Geometry: final body of the model. Coordinates: model frame, mm. A direction names the side the tool comes from. Give positions to 0.01 mm unless a question says otherwise; leave off trailing zeros. Loops run counter-clockwise (first coordinate to the right, second up) from the corner with the lowest first, then second, coordinate; pieces in that order, holes last.
```python
from build123d import *

# Parameters (mm, degrees)
CROQUIS2_R              = 6.5
SALIENTE_EXTRUIR1_DEPTH = 3
CROQUIS3_R              = 3
SALIENTE_EXTRUIR2_DEPTH = 70
CROQUIS4_OUTSIDE_W      = 32.968
CROQUIS4_OUTSIDE_H      = 32.968
CROQUIS4_OUTSIDE_R      = 6.25
CORTAR_EXTRUIR1_DEPTH   = 4
CORTAR_EXTRUIR1_DRAFT   = -20
CROQUIS6_W              = 1.6
CROQUIS6_H              = 14.093492938
CORTAR_EXTRUIR2_DEPTH   = 1.7


# Read off the part's stored shape, not the designer's step: #12-24 Machine Threads Stud1
with BuildPart() as part:
    # Croquis2 → Saliente-Extruir1 (new body)
    with BuildSketch(Plane.XY):
        Circle(CROQUIS2_R)
    extrude(amount=SALIENTE_EXTRUIR1_DEPTH)

    # Croquis3 → Saliente-Extruir2 (add)
    with BuildSketch(Plane(origin=(0, 0, 0), x_dir=(-1, 0, 0), z_dir=(0, 0, -1))):
        Circle(CROQUIS3_R)
    extrude(amount=SALIENTE_EXTRUIR2_DEPTH)


with BuildPart() as cortar_extruir1_tool:
    # Croquis4 outside → Cortar-Extruir1 (with draft: the straight prism first)
    with BuildSketch(Plane.XY.offset(3)):
        Rectangle(CROQUIS4_OUTSIDE_W, CROQUIS4_OUTSIDE_H)
        Circle(CROQUIS4_OUTSIDE_R, mode=Mode.SUBTRACT)
    extrude(amount=-CORTAR_EXTRUIR1_DEPTH)
    # Cortar-Extruir1: the draft: its side faces are tilted about the plane it starts from
    cortar_extruir1_sides = [cortar_extruir1_tool.faces().sort_by_distance(p)[0] for p in [
        (0, -16.484, 1),
        (16.484, 0, 1),
        (0, 16.484, 1),
        (-16.484, 0, 1),
        (-6.25, 0, 1),
    ]]
    draft(cortar_extruir1_sides, Plane.XY.offset(3), CORTAR_EXTRUIR1_DRAFT)


with BuildPart() as part_1:
    add(part.part)

    # Cortar-Extruir1: cut by cortar_extruir1_tool
    add(cortar_extruir1_tool.part, mode=Mode.SUBTRACT)

    # Croquis6 → Cortar-Extruir2 (cut)
    with BuildSketch(Plane.XY.offset(3)):
        Rectangle(CROQUIS6_W, CROQUIS6_H)
    extrude(amount=-CORTAR_EXTRUIR2_DEPTH, mode=Mode.SUBTRACT)

    # #12-24 Machine Threads Stud1 outline → #12-24 Machine Threads Stud1 (revolve, cut)
    with BuildSketch(Plane.XZ):
        with BuildLine():
            Line((2.11328, -70), (3, -70))
            Line((3, -70), (3, -57.153588301))
            Line((3, -57.153588301), (2.543199892, -57.153588301))
            ThreePointArc((2.543199892, -57.153588301), (2.118935595, -57.329324327), (1.943199568, -57.753588625))
            Line((1.943199568, -57.753588625), (1.943199568, -58.453589003))
            ThreePointArc((1.943199568, -58.453589003), (1.963644083, -58.608880514), (2.023584369, -58.753589165))
            Line((2.023584369, -58.753589165), (2.7432, -60))
            Line((2.7432, -60), (2.7432, -69.37008))
            Line((2.7432, -69.37008), (2.11328, -70))
        make_face()
    revolve(axis=Axis((0, 0, 0), (0, 0, 1)), mode=Mode.SUBTRACT)


solid = part_1.part
```
Q1. Section query B-B, the plane x = 0. Return loops of the section in (y, z), and give its area (3 significant figures).
Q2. Section query D-D, the plane z = -35.5. Return loops of the section in (x, y).
Q3. Section query C-C, the plane z = -62.5. Return loops of the section in (x, y), and give its area (3 significant figures).
Q4. Mould query, pull axis Z, two halves, no side actions, for faces 1 (the face through (0, 0, -70)), 2 (the face through (-1.432, 1.313, -58.108)), 3 (the face through (-0.8, 0, 2)). Classes: +Z half, -Z half, draft (parallel to the pull), parting line (faces both ways), or undercut.
Q5. Pin query (flat end, axial travel): pin 1 Ø6 at (x, y) = (3, -4) entering from -Z; pin 2 Ø1.4 at (y, z) = (-2, 2.5) entering from +X; pin 3 Ø3 at (y, z) = (1.5, -35.5) entering from +X; pin 4 Ø1.4 at (y, z) = (2, 2) entering from -X. Return the tip coordinate at first contact, or that it passes through.
Q6. Reachability of faces 4 (the face through (0, 0, 1.3)), 5 (the face through (3, -1, 0)), 6 (the face through (6.316, -0.128, 2.814)) from +Z, -Z, +X, -X, +Y, -Y: full face, straight path, thin tool, end or side. Return the list, or none.
Q7. Material intervals for probe 1 along Z at (x, y) = (3.5, -4); probe 2 along Z at (x, y) = (1.75, 2.25); probe 3 along X at (y, z) = (1.5, -39), sorted ascending.
Q8. Section query A-A, the plane y = 0. Return loops of the section in (x, z).
Resolved:
1. outline: (-6.5, 0) - (-3, 0) - (-3, -57.15) - (-2.54, -57.15) arc R0.6 cw to (-1.94, -57.75) - (-1.94, -58.45) arc R0.6 cw to (-2.02, -58.75) - (-2.74, -60) - (-2.74, -69.37) - (-2.11, -70) - (2.11, -70) - (2.74, -69.37) - (2.74, -60) - (2.02, -58.75) arc R0.6 cw to (1.94, -58.45) - (1.94, -57.75) arc R0.6 cw to (2.54, -57.15) - (3, -57.15) - (3, 0) - (6.5, 0) - (6.5, 1.3) - (-6.5, 1.3) - close
1. area: 427 mm2
2. outline: circle Ø6 at (0, 0)
3. outline: circle Ø5.49 at (0, 0)
3. area: 23.6 mm2
4. face 1: -Z half
4. face 2: undercut
4. face 3: draft
5. pin 1: stops at z = -70
5. pin 2: stops at x = 6.36
5. pin 3: stops at x = 3
5. pin 4: stops at x = -6.37
6. face 4: +Z, +Y, -Y
6. face 5: -Z
6. face 6: +Z, +X
7. probe 1: z = 0 to 3
7. probe 2: z = -57.15 to 3
7. probe 3: x = -2.6 to 2.6
8. outline: (-6.5, 0) - (-3, 0) - (-3, -57.15) - (-2.54, -57.15) arc R0.6 cw to (-1.94, -57.75) - (-1.94, -58.45) arc R0.6 cw to (-2.02, -58.75) - (-2.74, -60) - (-2.74, -69.37) - (-2.11, -70) - (2.11, -70) - (2.74, -69.37) - (2.74, -60) - (2.02, -58.75) arc R0.6 cw to (1.94, -58.45) - (1.94, -57.75) arc R0.6 cw to (2.54, -57.15) - (3, -57.15) - (3, 0) - (6.5, 0) - (6.5, 2.31) - (6.25, 3) - (0.8, 3) - (0.8, 1.3) - (-0.8, 1.3) - (-0.8, 3) - (-6.25, 3) - (-6.5, 2.31) - close
